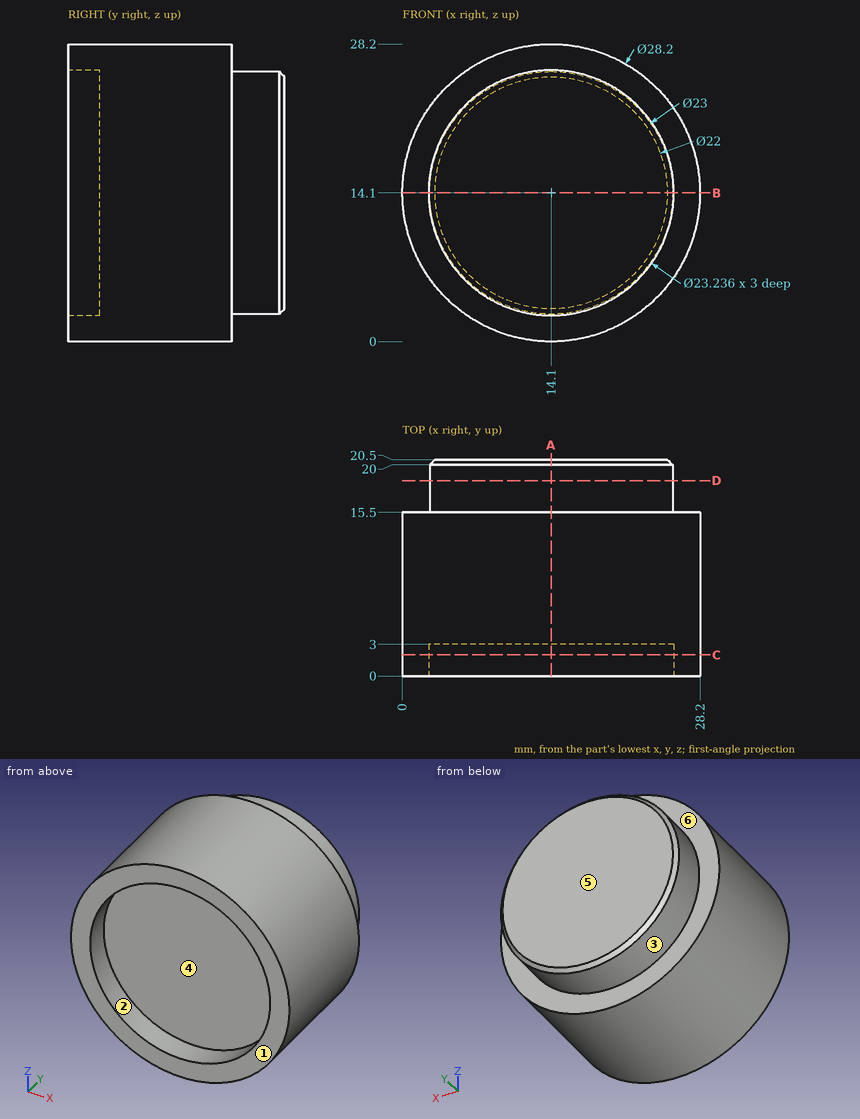
Check sheet for the drawn part. Datum: minimum x, y, z corner. Units: mm. A direction names the side the tool comes from. Give positions to 0.01 mm unless a question says otherwise; leave off trailing zeros. Write each loop counter-clockwise with the first axis right and the second up, starting at its lowest first coordinate (ties: lowest second). Pieces come first, ordered by that corner, then holes. Notation, with made-up numbers: (70.25, 59) -> (104.25, 59) arc R26 cw to (104.25, 96) -> close; hole circle Ø5 at (27, 45.25). An arc over 180 degrees is marked (long way). Use one line per item in the form item = value. Start each with the question number.
1. Section check A-A (x = 14.1). Record the cut outline in (y, z).
2. Go/stop test with flat-tipped pins: P1, Ø14, axis at x = 14.1, z = 14.1, coming from the -Y side; P2, Ø10, axis at y = 16, z = 5.5, coming from the -X side; P3, Ø3, axis at x = 11, y = 7.5, coming from the +Z side. Record where each tip stops, or that it passes through.
3. Thickness scan on line 1 along X through (y, z) = (2, 14.1); line 2 along Y through (x, z) = (27, 10); line 3 along Y through (x, z) = (22.5, 7.5). Record the ranges inside material, lowest first. Write a range as from..to.
4. Mould release check, pull along X, two halves, no side actions. Record for the marked faces 1, 2 and 3: pulls with the +X half, pulls with the -X half, needs draft (parallel to the pull), parting line crosses it, or undercut.
5. Section check D-D (y = 18.5). Record the cut outline in (x, z), and give its area (3 significant figures).
6. Section check B-B (z = 14.1). Record the cut outline in (x, y).
7. Section check C-C (y = 2). Record the cut outline in (x, z), and give its area (3 significant figures).
8. Access from +Z, -Z, +X, -X, +Y, -Y to the whole of each face (thin tool, end or side, straight path). Record for the marked faces 4, 5 and 6.
Conclusion:
q1.outline = (0, 0) -> (15.5, 0) -> (15.5, 2.6) -> (20, 2.6) -> (20.5, 3.1) -> (20.5, 25.1) -> (20, 25.6) -> (15.5, 25.6) -> (15.5, 28.2) -> (0, 28.2) -> (0, 25.72) -> (3, 25.72) -> (3, 2.48) -> (0, 2.48) -> close
q2.P1 = 3
q2.P2 = 0.47
q2.P3 = 28.11
q3.line_1 = 0..2.48, 25.72..28.2
q3.line_2 = 0..15.5
q3.line_3 = 3..20.5
q4.face_1 = needs draft
q4.face_2 = undercut
q4.face_3 = parting line crosses it
q5.outline = circle Ø23 at (14.1, 14.1)
q5.area = 415 mm²
q6.outline = (0, 0) -> (2.48, 0) -> (2.48, 3) -> (25.72, 3) -> (25.72, 0) -> (28.2, 0) -> (28.2, 15.5) -> (25.6, 15.5) -> (25.6, 20) -> (25.1, 20.5) -> (3.1, 20.5) -> (2.6, 20) -> (2.6, 15.5) -> (0, 15.5) -> close
q7.outline = circle Ø28.2 at (14.1, 14.1); hole circle Ø23.24 at (14.1, 14.1)
q7.area = 201 mm²
q8.face_4 = -Y
q8.face_5 = +Z, -Z, +X, -X, +Y
q8.face_6 = +Y
